from build123d import *

# Parameters (mm, degrees)
TUBE043_R                 = 85
TUBE043_R_2               = 80
TUBE043_DEPTH             = 13
TUBE042_R                 = 100
TUBE042_R_2               = 80
TUBE042_DEPTH             = 200
PAD041_DEPTH              = 100
PAD042_DEPTH              = 2
COMMON020_PLACEMENT_ANGLE = 20
ARRAY017_COUNT            = 22
ARRAY017_PLACEMENT_ANGLE  = 180
TUBE044_R                 = 34
TUBE044_R_2               = 30
TUBE044_DEPTH             = 13
PAD040_DEPTH              = 100


with BuildPart() as tube043:
    # Tube043 → Tube043 (new body)
    with BuildSketch(Plane.XY.offset(42.5)):
        Circle(TUBE043_R)
        Circle(TUBE043_R_2, mode=Mode.SUBTRACT)
    extrude(amount=TUBE043_DEPTH)


with BuildPart() as tube042:
    # Tube042 → Tube042 (new body)
    with BuildSketch(Plane.XY):
        Circle(TUBE042_R)
        Circle(TUBE042_R_2, mode=Mode.SUBTRACT)
    extrude(amount=TUBE042_DEPTH)


with BuildPart() as body042:
    # Sketch041 → Pad041 (new body)
    with BuildSketch(Plane.XZ):
        Polygon((0, 0), (0, 2), (26, 0.9), (26, 0), align=None)
    extrude(amount=PAD041_DEPTH)


with BuildPart() as body042_1:
    # Body042 placement: moved
    add(body042.part.moved(Location((-5, 0, 5))))


with BuildPart() as cut014:
    # Sketch042 → Pad042 (new body)
    with BuildSketch(Plane.XY):
        Polygon((0, 0), (0, -52), (25.94305, -47.924315), (8.5, 0), align=None)
    extrude(amount=PAD042_DEPTH)


with BuildPart() as cut014_1:
    # Body043 placement: moved
    add(cut014.part.moved(Location((-5, -33, 5))))

    # Common020: intersect Body042
    add(body042_1.part, mode=Mode.INTERSECT)


with BuildPart() as cut014_2:
    # Common020 placement: moved
    add(cut014_1.part.rotate(Axis((0, 0, 0), (0, 1, 0)), COMMON020_PLACEMENT_ANGLE))

    # Array017: Cut014 ×22 about axis
    array017_axis = Axis((0, 0, 0), (0, 0, 1))


with BuildPart() as cut014_3:
    add(cut014_2.part)
    for i in range(1, ARRAY017_COUNT):
        add(cut014_2.part.rotate(array017_axis, i * 360 / ARRAY017_COUNT))


with BuildPart() as cut014_4:
    # Array017 placement: moved
    add(cut014_3.part.moved(Location((0, 0, 52))).rotate(Axis((0, 0, 52), (0, 1, 0)), ARRAY017_PLACEMENT_ANGLE))

    # Cut014: cut Tube042
    add(tube042.part, mode=Mode.SUBTRACT)


with BuildPart() as pre3stat001:
    # Tube044 → Tube044 (new body)
    with BuildSketch(Plane.XY.offset(42.5)):
        Circle(TUBE044_R)
        Circle(TUBE044_R_2, mode=Mode.SUBTRACT)
    extrude(amount=TUBE044_DEPTH)

    # Fusion019: union Tube043, Cut014
    add(tube043.part)
    add(cut014_4.part)


with BuildPart() as stator3h1:
    # Sketch040 → Pad040 (new body)
    with BuildSketch(Plane.XY):
        Polygon((-6.733461, -90.278511), (6.859371, 102.08947), (-116.658012, 102.08947), (-116.658012, -85.846069), align=None)
    extrude(amount=PAD040_DEPTH)

    # Common021: intersect Pre3Stat001
    add(pre3stat001.part, mode=Mode.INTERSECT)


solid = stator3h1.part
Can you work these out from the model? Positions are in its coordinate system, mm. A direction names the side the tool comes from. Give positions to 0.01 mm unless a question says otherwise; leave off trailing zeros. Order: outer loops, then holes, each group sorted by start corner. A loop starts at its lowest first (then second) coordinate and runs counter-clockwise, first axis right, second up. Notation, with made-up numbers: M -26.75,-36.5 L 7.25,-36.5 A22 cw 7.25,-15.5 Z; hole C -11,3 d6. An arc over 180 degrees is marked long. Use one line per item in the form item = value. Start each with the question number.
Item 1: If I drill on line 1 along Y through (x, z) = (-0.5, 54.5); line 2 along Y through (x, z) = (-8, 54.25); line 3 along Y through (x, z) = (-11.5, 52), over which ranges is the centre line in solid material (lowest first)?
Item 2: For faces 1 (the flat face through (-18.49, 53.56, 44.66)), 2 (the flat face through (-50.661, -26.697, 50.747)), 3 (the cylindrical face through (-79.658, 7.387, 48.909)), which set-ups out of +Z, -Z, +X, -X, +Y, -Y let a thin tool reach every point of the face, with its end or its side?
Item 3: If we section it at C-C (x = 0): Write out the boundary of the cut face in (y, z).
Item 4: Will these pins go through, and if not, where does the flat tip stop? pin 1 Ø1.5 at (x, z) = (-69, 53) entering from +Y; pin 2 Ø6 at (x, z) = (-60, 49) entering from -Y; pin 3 Ø6 at (y, z) = (-25, 50) entering from -X.
Item 5: If we section it at A-A (y = -57): Write out the boundary of the cut face in (x, z), then the cut area to 3 significant figures.
Item 6: If we section it at B-B (y = 44.5): Write out the boundary of the cut face in (x, z).
Item 7: We'd pull the mould along Z, two halves only. Please class faces 4 (the flat face through (-44.51, 35.06, 44.66)), 5 (the flat face through (3.69, 57.25, 47.04)), 6 (the flat face through (-28.185, -49.848, 50.747)): +Z half, -Z half, draft (parallel to the pull), parting line (faces both ways), or undercut.
Outcome:
q1.line_1 = 30 to 34, 80 to 85
q1.line_2 = -84.62 to -79.6, -33.05 to -28.91, 28.91 to 33.05, 79.6 to 84.62
q1.line_3 = -84.22 to -79.17, -32 to -27.71, 27.71 to 32, 79.17 to 84.22
q2.face_1 = -Z
q2.face_2 = +Z
q2.face_3 = none
q3.outline = M 30,42.5 L 34,42.5 L 34,44.66 L 80,44.66 L 80,42.5 L 85,42.5 L 85,55.5 L 80,55.5 L 80,46.68 L 34,46.68 L 34,55.5 L 30,55.5 Z
q4.pin_1 = 50.66
q4.pin_2 = -63.06
q4.pin_3 = -82.1
q5.outline = M -63.06,42.5 L -56.13,42.5 L -56.13,51.43 L -33.89,43.71 L -33.08,45.59 L -56.13,52.65 L -56.13,55.5 L -63.06,55.5 Z; M -33.45,51.28 L -14.34,43.71 L -13.62,45.59 L -32.99,52.36 Z; M -13.64,50.29 L -4.38,46.47 L -4.38,48.27 L -13.21,51.49 Z
q5.area = 175 mm2
q6.outline = M -72.42,42.5 L -66.48,42.5 L -66.48,49.97 L -55.15,51.91 L -55.67,53 L -66.48,51.36 L -66.48,55.5 L -72.42,55.5 Z; M -55.92,45.59 L -54.87,43.71 L -32.3,49.81 L -32.79,51.1 Z; M -32.15,45.59 L -31.34,43.71 L -16.62,48.82 L -17.1,50.2 Z; M -16.18,45.59 L -15.47,43.71 L -3.52,48.44 L -4,49.85 Z; M -2.99,45.59 L -2.3,43.71 L 2.79,45.81 L 2.79,47.69 Z
q7.face_4 = -Z half
q7.face_5 = draft
q7.face_6 = +Z half
